Input: part model. Units: mm. Frame: model coordinates. A direction names the side the tool comes from. Round coordinates to 2 decimals unless told otherwise and drop trailing zeros. Loops run counter-clockwise (first coordinate to the right, second up) from the corner with the lowest first, then second, coordinate; pieces in that order, holes last. Notation, with made-up numbers: (63.5, 57) -> (68.5, 57) arc R23 ccw to (68.5, 83) -> close; hole circle Ø8 at (31.25, 38). An arc over 180 degrees is marked (long way). Answer as a JSON object with one key per item and string values.
```python
from build123d import *

# Parameters (mm, degrees)
SCHIZZO1_W                   = 30
SCHIZZO1_H                   = 40
ESTRUSIONE_ESTRUSIONE1_DEPTH = 30
SMUSSO1_SIZE                 = 20
ESTRUSIONE_ESTRUSIONE2_DEPTH = 20
FORO_PER_VITE_M5_1_D         = 5.5
FORO_PER_VITE_M5_1_DEPTH     = 13
FORO_PER_VITE_M5_1_TIP       = 1.652366702
FORO_PER_VITE_M5_2_D         = 5.5
FORO_PER_VITE_M5_2_DEPTH     = 13
FORO_PER_VITE_M5_2_TIP       = 1.652366702
SCHIZZO6_W                   = 30
SCHIZZO6_H                   = 30
TAGLIO_ESTRUSIONE1_DEPTH     = 10


with BuildPart() as part:
    # Schizzo1 → Estrusione-Estrusione1 (new body)
    with BuildSketch(Plane.XY):
        with Locations((15, 20)):
            Rectangle(SCHIZZO1_W, SCHIZZO1_H)
    extrude(amount=ESTRUSIONE_ESTRUSIONE1_DEPTH)

    # Smusso1
    smusso1_edges = [part.edges().sort_by_distance(p)[0] for p in [
        (30, 20, 30),
        (30, 0, 15),
        (15, 0, 30),
    ]]
    chamfer(smusso1_edges, length=SMUSSO1_SIZE)

    # Schizzo2 → Estrusione-Estrusione2 (add)
    with BuildSketch(Plane(origin=(0, 40, 0), x_dir=(1, 0, 0), z_dir=(0, 1, 0))):
        Polygon((0, 0), (30, 0), (30, -10), (10, -30), (0, -30), align=None)
    extrude(amount=ESTRUSIONE_ESTRUSIONE2_DEPTH)

    # Foro per Vite M5-1
    with Locations(Plane.ZY):
        with Locations((18, 20), (18, 48)):
            Hole(FORO_PER_VITE_M5_1_D / 2, depth=FORO_PER_VITE_M5_1_DEPTH)
            with Locations((0, 0, -(FORO_PER_VITE_M5_1_DEPTH + FORO_PER_VITE_M5_1_TIP / 2))):  # 118° drill point
                Cone(0, FORO_PER_VITE_M5_1_D / 2, FORO_PER_VITE_M5_1_TIP, mode=Mode.SUBTRACT)

    # Foro per Vite M5-2
    with Locations(Plane(origin=(18, 20, 0), x_dir=(-1, 0, 0), z_dir=(0, 0, -1))):
        with Locations((0, 0), (0, 28)):
            Hole(FORO_PER_VITE_M5_2_D / 2, depth=FORO_PER_VITE_M5_2_DEPTH)
            with Locations((0, 0, -(FORO_PER_VITE_M5_2_DEPTH + FORO_PER_VITE_M5_2_TIP / 2))):  # 118° drill point
                Cone(0, FORO_PER_VITE_M5_2_D / 2, FORO_PER_VITE_M5_2_TIP, mode=Mode.SUBTRACT)

    # Schizzo6 → Taglio-Estrusione1 (cut)
    with BuildSketch(Plane.XZ):
        with Locations((15, 15)):
            Rectangle(SCHIZZO6_W, SCHIZZO6_H)
    extrude(amount=-TAGLIO_ESTRUSIONE1_DEPTH, mode=Mode.SUBTRACT)


solid = part.part
```
1) Reachability of faces 4 (the face through (10, 10, 10)), 5 (the face through (6.591, 20.121, 20.747)), 6 (the face through (17.642, 50.727, 6.591)) from +Z, -Z, +X, -X, +Y, -Y: full face, straight path, thin tool, end or side. Return the list, or none.
Output:
{"face 4": "+Z, -Z, +X, -X, -Y", "face 5": "-X", "face 6": "-Z"}
2) Section B-B, the plane x = 21.5. Output: boundary loops of the cut face in (y, z), plus the area to 3 significant figures.
Output:
{"outline": "(11.5, 0) -> (60, 0) -> (60, 18.5) -> (20, 18.5) -> (11.5, 10) -> close", "area": "861 mm^2"}
3) Draft query along Z for faces 1 (the face through (18, 16, 18)), 2 (the face through (17.743, 20.403, 14.365)), 3 (the face through (14.365, 20.323, 17.648)). Return one class per face: +Z half, -Z half, draft (parallel to the pull), parting line (faces both ways), or undercut.
Output:
{"face 1": "+Z half", "face 2": "-Z half", "face 3": "undercut"}
4) Section C-C, the plane y = 25. Output: boundary loops of the cut face in (x, z).
Output:
{"outline": "(0, 0) -> (30, 0) -> (30, 10) -> (10, 30) -> (0, 30) -> close"}
5) Contact query for flat-ended pins moving along their axis: P1, Ø7, axis at x = 18, y = 20, coming from the +Z side; P2, Ø6.5, axis at y = 48, z = 18, coming from the +X side; P3, Ø4.5, axis at x = 18, y = 48, coming from the -Z side. Output: stop coordinate, or through.
Output:
{"P1": "stops at z = 25.5", "P2": "stops at x = 25.25", "P3": "stops at z = 13.3"}
6) Section A-A, the plane z = 5. Output: boundary loops of the cut face in (x, y).
Output:
{"outline": "(0, 10) -> (20, 10) -> (30, 20) -> (30, 60) -> (0, 60) -> close; hole circle Ø5.5 at (18, 20); hole circle Ø5.5 at (18, 48)"}
7) Ray query, probe 1 along Y at (x, z) = (18, 4); probe 2 along Z at (x, y) = (10, 48); probe 3 along X at (y, z) = (47.5, 2). Return the intervals inside material, ascending.
Output:
{"probe 1": "y = 10 to 17.25, 22.75 to 45.25, 50.75 to 60", "probe 2": "z = 0 to 15.25, 20.75 to 30", "probe 3": "x = 0 to 15.3, 20.7 to 30"}
